```python
from build123d import *

# Parameters (mm, degrees)
SKETCH1_R           = 1
BOSS_EXTRUDE3_DEPTH = 1.5


with BuildPart() as part:
    # Sketch1 → Boss-Extrude3 (new body)
    with BuildSketch(Plane(origin=(0, 0, 0), x_dir=(0, 0, -1), z_dir=(1, 0, 0))):
        with BuildLine():
            Line((6.7641026, 1.999999498), (2.83655563, 1.999999498))
            ThreePointArc((2.83655563, 1.999999498), (2.231030071, 2.20417364), (1.872769834, 2.733321904))
            Line((1.872769834, 2.733321904), (0.835129535, 6.483404419))
            ThreePointArc((0.835129535, 6.483404419), (-1.933413156, 8.051897856), (-3.501906514, 5.283355121))
            Line((-3.501906514, 5.283355121), (-2.168518496, 0.464427051))
            ThreePointArc((-2.168518496, 0.464427051), (-0.964537658, -1.313845406), (1.07041083, -1.999999498))
            Line((1.07041083, -1.999999498), (6.7641026, -1.999999498))
            ThreePointArc((6.7641026, -1.999999498), (8.063140814, -2.295836094), (9.105977, -3.124999686))
            ThreePointArc((9.105977, -3.124999686), (18.009101, 0), (9.105977, 3.124999686))
            ThreePointArc((9.105977, 3.124999686), (8.063140814, 2.295836094), (6.7641026, 1.999999498))
        make_face()
        with Locations((-1.333388507, 5.883379832)):
            Circle(SKETCH1_R, mode=Mode.SUBTRACT)
        with Locations((0, 1.064451)):
            Circle(SKETCH1_R, mode=Mode.SUBTRACT)
        with BuildLine():
            Line((10.525768, 1.683168801), (10.525768, -1.683168801))
            ThreePointArc((10.525768, -1.683168801), (13.009101, -3), (15.492434, -1.683168801))
            Line((15.492434, -1.683168801), (15.492434, 1.683168801))
            ThreePointArc((15.492434, 1.683168801), (13.009101, 3), (10.525768, 1.683168801))
        make_face(mode=Mode.SUBTRACT)
    extrude(amount=BOSS_EXTRUDE3_DEPTH)


solid = part.part
```
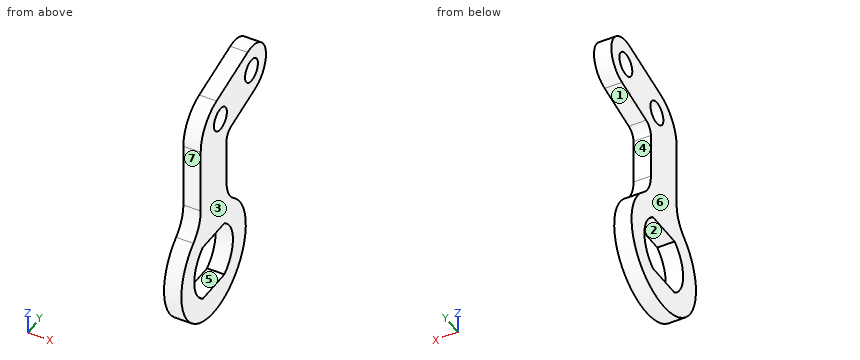
The model under review builds one solid part; all positions refer to its coordinate system, in mm. Face numbers are marked on the shaded views. A direction names the side the tool comes from. Give positions to 0.01 mm unless a question says otherwise; leave off trailing zeros. Write each loop counter-clockwise with the first axis right and the second up, starting at its lowest first coordinate (ties: lowest second). Pieces come first, ordered by that corner, then holes. Notation, with made-up numbers: M 48.5,49 L 80.5,49 A23 ccw 80.5,81 Z; hole C -37,24.5 d6. An arc over 180 degrees is marked long. Write each question's results on one line, items separated by ' | '. Start each with the question number.
1. We need section C-C (x = 0.95). Write out the cut boundary in (y, z) (3 decimals).
2. For probe 1 along Y at (x, z) = (1.2, -13); probe 2 along Y at (x, z) = (0.3, -6.25); probe 3 along Z at (x, y) = (0.95, 2.25), list the stretches that pass through material, from the lowest coordinate up. Write a range as [from, to].
3. For the marked faces 1, 2 and 3, list the 3-axis set-ups (+Z, -Z, +X, -X, +Y, -Y) from which the entire face can be reached by the end or side of a thin tool; tool diameter is ignored.
4. We need section D-D (z = -1.5). Write out the cut boundary in (x, y).
5. Insertion check: pin 1 Ø0.8 at (x, z) = (0.5, -2.5) entering from -Y; pin 2 Ø1.6 at (y, z) = (1.06, 0) entering from -X. Each pin has a flat end and moves straight along its axis. Give the tip position at first contact, or say it passes through.
6. We need section B-B (y = 3.5). Write out the cut boundary in (x, z).
7. Mouldability with a two-part tool opening along Y and no side actions: class the marked faces 4, 5, 6 and 7 as released by +Y, released by -Y, zero draft, split by the parting line, or undercut.
8. We need section A-A (z = -15.25). Write out the cut boundary in (x, y).
Results found:
1) outline: M -3.125,-9.106 A5 ccw long 3.125,-9.106 A3 cw 2,-6.764 L 2,-2.837 A1 cw 2.733,-1.873 L 6.483,-0.835 A2.25 ccw 5.283,3.502 L 0.464,2.169 A3.361 ccw -2,-1.07 L -2,-6.764 A3 cw Z; hole M -1.683,-15.492 L 1.683,-15.492 A3 ccw 1.683,-10.526 L -1.683,-10.526 A3 ccw Z; hole C 1.064,0 d2; hole C 5.883,1.333 d2
2) probe 1: y = [-5, -3], [3, 5] | probe 2: y = [-2, 2] | probe 3: z = [-17.47, -14.99], [-11.02, -7.96], [-2.18, 2.66]
3) face 1: +X, -X, +Y | face 2: +X, -X | face 3: +Z, -Z, +X, +Y, -Y
4) outline: M 0,-2 L 1.5,-2 L 1.5,4.08 L 0,4.08 Z
5) pin 1: stops at y = -2 | pin 2: passes through
6) outline: M 0,-16.58 L 1.5,-16.58 L 1.5,-9.44 L 0,-9.44 Z; M 0,-1.66 L 1.5,-1.66 L 1.5,3.01 L 0,3.01 Z
7) face 4: released by +Y | face 5: undercut | face 6: zero draft | face 7: released by -Y
8) outline: M 0,-4.47 L 1.5,-4.47 L 1.5,-1.99 L 0,-1.99 Z; M 0,1.99 L 1.5,1.99 L 1.5,4.47 L 0,4.47 Z
